Source: CAD feature listing. Evaluate the final solid. Frame: model axes, mm. A direction names the side the tool comes from. Give positions to 0.01 mm unless a question says otherwise; leave off trailing zeros. Write each loop counter-clockwise with the first axis right and the second up, starting at its lowest first coordinate (ties: lowest second). Pieces come first, ordered by that corner, then holes. Notation, with made-up numbers: (71.25, 58.5) - (100.25, 58.5) arc R18 cw to (100.25, 78.5) - close; hole circle Ø6 at (16.25, 61). An arc over 180 degrees is marked (long way). One line per question, with ' | ' between items. Start each with the question number.
(1) Pin query (flat end, axial travel): pin 1 (0.9 mm diameter, centred on x = -24.5, z = 1, fed in from -Y). Return the tip coordinate at first contact, or that it passes through.
(2) Section C-C, the plane x = -15.5. Return loops of the section in (y, z).
(3) Section D-D, the plane y = 7.5. Return loops of the section in (x, z), plus the area to 3 significant figures.
(4) Ray query, line 1 (X direction, y = -1.5, z = 2.55); line 2 (Y direction, x = -25, z = 1.75); line 3 (Y direction, x = 4, z = 2.3). Return the intervals inside material, ascending. Write a range as [from, to].
(5) Access query for faces 5 (the cylindrical face through (5.699, -6.715, 1.521)), 6 (the flat face through (7, -15.1, 1)). Directions: +Z, -Z, +X, -X, +Y, -Y. A direction counts if a zero-diameter tool reaches every point of the face in a straight line with its end or side. Return the directions, or none.
(6) Section A-A, the plane y = 0. Return loops of the section in (x, z), plus the area to 3 significant figures.
(7) Section B-B, the plane x = -29.05. Return loops of the section in (y, z).
(8) Draft query along X for faces 1 (the flat face through (-13, -15.1, 1)), 2 (the cylindrical face through (-29.07, 12.15, 1.48)), 3 (the cylindrical face through (9.699, -14.815, 1.521)), 4 (the flat face through (-30.1, -14, 1)). Return one class per face: +X half, -X half, draft (parallel to the pull), parting line (faces both ways), or undercut.
```python
from build123d import *

# Parameters (mm, degrees)
SKETCH_1_W      = 16.05
SKETCH_1_H      = 10
EXTRUDE_1_DEPTH = 3
FILLET_1_R      = 1


with BuildPart() as part:
    # 草图1 → 凸台-拉伸1 (new body)
    with BuildSketch(Plane.XY):
        with BuildLine():
            Line((-5.1, -15.1), (-5.1, -12))
            ThreePointArc((-5.1, -12), (-4.05, -10.95), (-3, -12))
            Line((-3, -12), (3, -12))
            ThreePointArc((3, -12), (4.05, -10.95), (5.1, -12))
            Line((5.1, -12), (5.1, -15.1))
            Line((5.1, -15.1), (10, -15.1))
            Line((10, -15.1), (10, 15.1))
            Line((10, 15.1), (-35.1, 15.1))
            Line((-35.1, 15.1), (-35.1, -15.1))
            Line((-35.1, -15.1), (-30.1, -15.1))
            Line((-30.1, -15.1), (-30.1, -12))
            ThreePointArc((-30.1, -12), (-29.05, -10.95), (-28, -12))
            Line((-28, -12), (-22, -12))
            ThreePointArc((-22, -12), (-20.95, -10.95), (-19.9, -12))
            Line((-19.9, -12), (-19.9, -15.1))
            Line((-19.9, -15.1), (-5.1, -15.1))
        make_face()
        with Locations((-2.025, -2)):
            Rectangle(SKETCH_1_W, SKETCH_1_H, mode=Mode.SUBTRACT)
        with BuildLine():
            Line((3, 8), (-3, 8))
            ThreePointArc((-3, 8), (-4.05, 6.95), (-5.1, 8))
            Line((-5.1, 8), (-5.1, 11.1))
            ThreePointArc((-5.1, 11.1), (-4.05, 12.15), (-3, 11.1))
            Line((-3, 11.1), (3, 11.1))
            ThreePointArc((3, 11.1), (4.05, 12.15), (5.1, 11.1))
            Line((5.1, 11.1), (5.1, 8))
            ThreePointArc((5.1, 8), (4.05, 6.95), (3, 8))
        make_face(mode=Mode.SUBTRACT)
        with BuildLine():
            ThreePointArc((-30.1, 11.1), (-29.05, 12.15), (-28, 11.1))
            Line((-28, 11.1), (-22, 11.1))
            ThreePointArc((-22, 11.1), (-20.95, 12.15), (-19.9, 11.1))
            Line((-19.9, 11.1), (-19.9, 8))
            ThreePointArc((-19.9, 8), (-20.95, 6.95), (-22, 8))
            Line((-22, 8), (-28, 8))
            ThreePointArc((-28, 8), (-29.05, 6.95), (-30.1, 8))
            Line((-30.1, 8), (-30.1, 11.1))
        make_face(mode=Mode.SUBTRACT)
        with Locations((-23.075, -2)):
            Rectangle(SKETCH_1_W, SKETCH_1_H, mode=Mode.SUBTRACT)
    extrude(amount=EXTRUDE_1_DEPTH)

    # 圆角1
    fillet_1_edges = [part.edges().sort_by_distance(p)[0] for p in [
        (6, -7, 1.5),
        (6, 3, 1.5),
        (-10.05, 3, 1.5),
        (-10.05, -7, 1.5),
        (10, 15.1, 1.5),
        (10, -15.1, 1.5),
    ]]
    fillet(fillet_1_edges, radius=FILLET_1_R)


solid = part.part
```
Check sheet entries:
1) pin 1: y = -12
2) outline: (-15.1, 0) - (-7, 0) - (-7, 3) - (-15.1, 3) - close; (3, 0) - (15.1, 0) - (15.1, 3) - (3, 3) - close
3) outline: (-35.1, 0) - (-29.97, 0) - (-29.97, 3) - (-35.1, 3) - close; (-28.13, 0) - (-21.87, 0) - (-21.87, 3) - (-28.13, 3) - close; (-20.03, 0) - (-4.97, 0) - (-4.97, 3) - (-20.03, 3) - close; (-3.13, 0) - (3.13, 0) - (3.13, 3) - (-3.13, 3) - close; (4.97, 0) - (10, 0) - (10, 3) - (4.97, 3) - close | area: 113 mm²
4) line 1: [-35.1, -31.1], [-15.05, -10.05], [6, 10] | line 2: [-12, -7], [3, 8], [11.1, 15.1] | line 3: [-10.95, -7], [3, 6.95], [12.15, 15.1]
5) face 5: +Z, -Z | face 6: +Z, -Z, +X, -X, -Y
6) outline: (-35.1, 0) - (-31.1, 0) - (-31.1, 3) - (-35.1, 3) - close; (-15.05, 0) - (-10.05, 0) - (-10.05, 3) - (-15.05, 3) - close; (6, 0) - (10, 0) - (10, 3) - (6, 3) - close | area: 39.0 mm²
7) outline: (-10.95, 0) - (-7, 0) - (-7, 3) - (-10.95, 3) - close; (3, 0) - (6.95, 0) - (6.95, 3) - (3, 3) - close; (12.15, 0) - (15.1, 0) - (15.1, 3) - (12.15, 3) - close
8) face 1: draft | face 2: undercut | face 3: +X half | face 4: undercut
